Input: part model. Units: mm. Frame: model coordinates. A direction names the side the tool comes from. Coordinates: 2 decimals unless noted, no trailing zeros. Write each loop counter-clockwise with the first axis right and the second up, starting at its lowest first coordinate (ties: lowest second). Pieces come first, ordered by that corner, then holes. Notation, with made-up numbers: (-28.75, 49) - (7.25, 49) arc R24 cw to (7.25, 78) - close; hole circle Ø8 at (53.5, 5). An arc over 180 degrees is marked (long way). Use a Markdown table: item, result. Add a question column.
Q1. Section query C-C (z = 32). Return the cut outline in (x, y), then the cut area to 3 significant figures.
Q2. Material intervals for probe 1 along Z at (x, y) = (-21.5, 6); probe 2 along Z at (x, y) = (13.5, -10.5); probe 3 along Y at (x, z) = (0, 17.5), sorted ascending. Write a range as from..to.
Q3. Section query A-A (x = 0). Return the cut outline in (y, z).
Q4. Set-up query: faces 1 (the face through (5, -11, 0)), 2 (the face through (-14.985, 0.66, 8.916)), 3 (the face through (-11, 17, 18)). Return all of +Z, -Z, +X, -X, +Y, -Y with unobstructed straight access to the full face (end or side cutting, diameter ignored); none if empty.
Q5. Mould query, pull axis Y, two halves, no side actions, for faces 4 (the face through (-2.38, -10.74, 19.27)), 5 (the face through (9, -9, 38)), 6 (the face through (-4.336, -19.524, 27.86)). Classes: released by +Y, released by -Y, zero draft, split by the parting line, or undercut.
Q6. Pin query (flat end, axial travel): P1, Ø2, axis at y = -18, z = 28, coming from the +X side; P2, Ø4, axis at y = 5, z = 16.5, coming from the +X side; P3, Ø12, axis at y = -13.5, z = 14.5, coming from the -X side; P4, Ø20, axis at x = 0, y = 0, coming from the -Z side. Return the tip coordinate at first contact, or that it passes through.
Q7. Section query D-D (y = -14). Return the cut outline in (x, z), then the cut area to 3 significant figures.
from build123d import *

# Parameters (mm, degrees)
SKETCH1_R           = 25
BOSS_EXTRUDE1_DEPTH = 3
SKETCH2_R           = 15
BOSS_EXTRUDE2_DEPTH = 15
SKETCH3_R           = 25
BOSS_EXTRUDE3_DEPTH = 3
SKETCH4_R           = 20
BOSS_EXTRUDE4_DEPTH = 20
SKETCH5_R           = 11
CUT_EXTRUDE1_DEPTH  = 50


with BuildPart() as part:
    # Sketch1 → Boss-Extrude1 (new body)
    with BuildSketch(Plane.XY):
        Circle(SKETCH1_R)
    extrude(amount=BOSS_EXTRUDE1_DEPTH)

    # Sketch2 → Boss-Extrude2 (add)
    with BuildSketch(Plane.XY):
        Circle(SKETCH2_R)
    extrude(amount=BOSS_EXTRUDE2_DEPTH)

    # Sketch3 → Boss-Extrude3 (add)
    with BuildSketch(Plane.XY.offset(15)):
        Circle(SKETCH3_R)
    extrude(amount=BOSS_EXTRUDE3_DEPTH)

    # Sketch4 → Boss-Extrude4 (add)
    with BuildSketch(Plane.XY.offset(18)):
        Circle(SKETCH4_R)
    extrude(amount=BOSS_EXTRUDE4_DEPTH)

    # Sketch5 → Cut-Extrude1 (cut)
    with BuildSketch(Plane.XY.offset(38)):
        Circle(SKETCH5_R)
    extrude(amount=-CUT_EXTRUDE1_DEPTH, mode=Mode.SUBTRACT)


solid = part.part
Values follow:
| question | item | result |
|---|---|---|
| 1 | outline | circle Ø40 at (0, 0); hole circle Ø22 at (0, 0) |
| 1 | area | 877 mm2 |
| 2 | probe 1 | 0..3, 15..18 |
| 2 | probe 2 | 0..3, 15..38 |
| 2 | probe 3 | -25..-11, 11..25 |
| 3 | outline | (-25, 0) - (-11, 0) - (-11, 38) - (-20, 38) - (-20, 18) - (-25, 18) - (-25, 15) - (-15, 15) - (-15, 3) - (-25, 3) - close; (11, 0) - (25, 0) - (25, 3) - (15, 3) - (15, 15) - (25, 15) - (25, 18) - (20, 18) - (20, 38) - (11, 38) - close |
| 4 | face 1 | -Z, +X, -X, +Y, -Y |
| 4 | face 2 | none |
| 4 | face 3 | +Z |
| 5 | face 4 | undercut |
| 5 | face 5 | zero draft |
| 5 | face 6 | split by the parting line |
| 6 | P1 | x = 10.54 |
| 6 | P2 | x = 24.82 |
| 6 | P3 | x = -23.84 |
| 6 | P4 | through |
| 7 | outline | (-20.71, 0) - (20.71, 0) - (20.71, 3) - (5.39, 3) - (5.39, 15) - (20.71, 15) - (20.71, 18) - (14.28, 18) - (14.28, 38) - (-14.28, 38) - (-14.28, 18) - (-20.71, 18) - (-20.71, 15) - (-5.39, 15) - (-5.39, 3) - (-20.71, 3) - close |
| 7 | area | 949 mm2 |
